```python
from build123d import *

# Parameters (mm, degrees)
SKETCH_1_W               = 135
SKETCH_1_H               = 100
EXTRUDE_1_DEPTH          = 4
SKETCH_2_W               = 135
SKETCH_2_H               = 4
EXTRUDE_2_DEPTH          = 60
CUT_EXTRUDE_1_DEPTH      = 130.12106722
CUT_EXTRUDE_1_DEPTH_BACK = 130.12106722
SKETCH_3_W               = 3
SKETCH_3_H               = 50
FILLET_1_R               = 5
FILLET_2_R               = 2
CUT_EXTRUDE_2_DEPTH      = 130.12106722
CUT_EXTRUDE_2_DEPTH_BACK = 130.12106722
SKETCH_4_R               = 1.75
CUT_EXTRUDE_3_DEPTH      = 130.12106722
CUT_EXTRUDE_3_DEPTH_BACK = 130.12106722
SKETCH_5_W               = 34
SKETCH_5_H               = 12
CUT_EXTRUDE_4_DEPTH      = 130.12106722
CUT_EXTRUDE_4_DEPTH_BACK = 130.12106722
SKETCH_6_R               = 1.75
SKETCH_7_W               = 48.5
SKETCH_7_H               = 4
CUT_EXTRUDE_5_DEPTH      = 22
CUT_EXTRUDE_6_DEPTH      = 130.12106722
CUT_EXTRUDE_6_DEPTH_BACK = 130.12106722
SKETCH_8_R               = 1.75
CUT_EXTRUDE_7_DEPTH      = 130.12106722
CUT_EXTRUDE_7_DEPTH_BACK = 130.12106722
SKETCH_9_R               = 1.75


with BuildPart() as part:
    # 草图1 → 凸台-拉伸1 (new body)
    with BuildSketch(Plane(origin=(0, 0, 0), x_dir=(1, 0, 0), z_dir=(0, 1, 0))):
        Rectangle(SKETCH_1_W, SKETCH_1_H)
    extrude(amount=EXTRUDE_1_DEPTH)

    # 草图2 → 凸台-拉伸2 (add)
    with BuildSketch(Plane.XY.offset(50)):
        with Locations((0, 2)):
            Rectangle(SKETCH_2_W, SKETCH_2_H)
    extrude(amount=EXTRUDE_2_DEPTH)

    # 草图3 → 切除-拉伸1 (cut, two sides: drawn at the far end of the back side and taken through both)
    with BuildSketch(Plane(origin=(0, 4, 0), x_dir=(1, 0, 0), z_dir=(0, 1, 0)).offset(-CUT_EXTRUDE_1_DEPTH_BACK)):
        with Locations((-66, 25)):
            Rectangle(SKETCH_3_W, SKETCH_3_H)
        with Locations((66, 25)):
            Rectangle(SKETCH_3_W, SKETCH_3_H)
        with Locations((-66, -85)):
            Rectangle(SKETCH_3_W, SKETCH_3_H)
        with Locations((66, -85)):
            Rectangle(SKETCH_3_W, SKETCH_3_H)
    extrude(amount=CUT_EXTRUDE_1_DEPTH + CUT_EXTRUDE_1_DEPTH_BACK, mode=Mode.SUBTRACT)

    # 圆角1
    fillet_1_edges = [part.edges().sort_by_distance(p)[0] for p in [
        (64.5, 2, -50),
        (-64.5, 2, 110),
        (64.5, 2, 110),
        (-64.5, 2, -50),
    ]]
    fillet(fillet_1_edges, radius=FILLET_1_R)

    # 圆角2
    fillet_2_edges = [part.edges().sort_by_distance(p)[0] for p in [
        (67.5, 2, 0),
        (-67.5, 2, 60),
        (67.5, 2, 60),
        (-67.5, 2, 0),
    ]]
    fillet(fillet_2_edges, radius=FILLET_2_R)

    # 草图4 → 切除-拉伸2 (cut, two sides: drawn at the far end of the back side and taken through both)
    with BuildSketch(Plane(origin=(0, 4, 0), x_dir=(1, 0, 0), z_dir=(0, 1, 0)).offset(-CUT_EXTRUDE_2_DEPTH_BACK)):
        with Locations(Location((-30, -102, 0), (0, 0, 270))):
            Circle(SKETCH_4_R)
        with Locations(Location((0, -102, 0), (0, 0, 270))):
            Circle(SKETCH_4_R)
        with Locations(Location((30, -102, 0), (0, 0, 270))):
            Circle(SKETCH_4_R)
        with Locations(Location((-30, 42, 0), (0, 0, 270))):
            Circle(SKETCH_4_R)
        with Locations(Location((0, 42, 0), (0, 0, 270))):
            Circle(SKETCH_4_R)
        with Locations(Location((30, 42, 0), (0, 0, 270))):
            Circle(SKETCH_4_R)
    extrude(amount=CUT_EXTRUDE_2_DEPTH + CUT_EXTRUDE_2_DEPTH_BACK, mode=Mode.SUBTRACT)

    # 草图5 → 切除-拉伸3 (cut, two sides: drawn at the far end of the back side and taken through both)
    with BuildSketch(Plane(origin=(0, 4, 0), x_dir=(1, 0, 0), z_dir=(0, 1, 0)).offset(-CUT_EXTRUDE_3_DEPTH_BACK)):
        with Locations((0, -86)):
            Rectangle(SKETCH_5_W, SKETCH_5_H)
        with Locations((0, 26)):
            Rectangle(SKETCH_5_W, SKETCH_5_H)
    extrude(amount=CUT_EXTRUDE_3_DEPTH + CUT_EXTRUDE_3_DEPTH_BACK, mode=Mode.SUBTRACT)

    # 草图6 → 切除-拉伸4 (cut, two sides: drawn at the far end of the back side and taken through both)
    with BuildSketch(Plane.XZ.offset(-CUT_EXTRUDE_4_DEPTH_BACK)):
        with Locations(Location((-16, -2, 0), (0, 0, 270))):
            Circle(SKETCH_6_R)
        with Locations(Location((16, -2, 0), (0, 0, 270))):
            Circle(SKETCH_6_R)
        with Locations(Location((16, 62, 0), (0, 0, 270))):
            Circle(SKETCH_6_R)
        with Locations(Location((-16, 62, 0), (0, 0, 270))):
            Circle(SKETCH_6_R)
    extrude(amount=CUT_EXTRUDE_4_DEPTH + CUT_EXTRUDE_4_DEPTH_BACK, mode=Mode.SUBTRACT)

    # 草图7 → 切除-拉伸5 (cut)
    with BuildSketch(Plane(origin=(0, 0, -50), x_dir=(-1, 0, 0), z_dir=(0, 0, -1))):
        with Locations((0, 2)):
            Rectangle(SKETCH_7_W, SKETCH_7_H)
    extrude(amount=-CUT_EXTRUDE_5_DEPTH, mode=Mode.SUBTRACT)

    # 草图8 → 切除-拉伸6 (cut, two sides: drawn at the far end of the back side and taken through both)
    with BuildSketch(Plane.XZ.offset(-CUT_EXTRUDE_6_DEPTH_BACK)):
        with Locations(Location((-29, -32.13, 0), (0, 0, 270))):
            Circle(SKETCH_8_R)
        with Locations(Location((29, -32.13, 0), (0, 0, 270))):
            Circle(SKETCH_8_R)
    extrude(amount=CUT_EXTRUDE_6_DEPTH + CUT_EXTRUDE_6_DEPTH_BACK, mode=Mode.SUBTRACT)

    # 草图9 → 切除-拉伸7 (cut, two sides: drawn at the far end of the back side and taken through both)
    with BuildSketch(Plane(origin=(0, 4, 0), x_dir=(1, 0, 0), z_dir=(0, 1, 0)).offset(-CUT_EXTRUDE_7_DEPTH_BACK)):
        with Locations(Location((-63, -30, 0), (0, 0, 270))):
            Circle(SKETCH_9_R)
        with Locations(Location((-63, -20, 0), (0, 0, 270))):
            Circle(SKETCH_9_R)
        with Locations(Location((-63, -10, 0), (0, 0, 270))):
            Circle(SKETCH_9_R)
        with Locations(Location((-63, -40, 0), (0, 0, 270))):
            Circle(SKETCH_9_R)
        with Locations(Location((-63, -50, 0), (0, 0, 270))):
            Circle(SKETCH_9_R)
        with Locations(Location((63, -50, 0), (0, 0, 270))):
            Circle(SKETCH_9_R)
        with Locations(Location((63, -40, 0), (0, 0, 270))):
            Circle(SKETCH_9_R)
        with Locations(Location((63, -30, 0), (0, 0, 270))):
            Circle(SKETCH_9_R)
        with Locations(Location((63, -20, 0), (0, 0, 270))):
            Circle(SKETCH_9_R)
        with Locations(Location((63, -10, 0), (0, 0, 270))):
            Circle(SKETCH_9_R)
    extrude(amount=CUT_EXTRUDE_7_DEPTH + CUT_EXTRUDE_7_DEPTH_BACK, mode=Mode.SUBTRACT)


solid = part.part
```
Could you check a few things on this model? Use its own coordinates, in mm. A direction names the side the tool comes from. Round coordinates to 2 decimals unless told otherwise and drop trailing zeros. Write each loop counter-clockwise with the first axis right and the second up, starting at its lowest first coordinate (ties: lowest second). Pieces come first, ordered by that corner, then holes. Notation, with made-up numbers: M -23.75,50.5 L -5.75,50.5 A27 ccw -5.75,76.5 Z; hole C 59,64.25 d4. An arc over 180 degrees is marked long. Answer in a Markdown table with one row per item. Add a question column.
Q1. Imagine slicing it at A-A (z = 10). Please give me the cut outline in (x, y).
Q2. Imagine slicing it at C-C (y = 3.25). Give the number of separate pieces and of enclosed holes in the cut face, then the cut area to 3 significant figures.
Q3. Will these pins go through, and if not, where does the flat tip stop? pin 1 Ø2 at (y, z) = (3.5, -11) entering from -X; pin 2 Ø2 at (x, y) = (3, 2.5) entering from -Z; pin 3 Ø10 at (x, z) = (-19, 8) entering from -Y; pin 4 Ø3 at (x, z) = (-63, 40) entering from -Y.
Q4. On a 3-axis mill with a long thin cutter (end or side, diameter ignored), from which of +Z, -Z, +X, -X, +Y, -Y can I reach the whole of each face in a straight line? I mean faces 1 (the flat face through (-17, 2, -24)), 2 (the flat face through (42, 2, -50)), 3 (the flat face through (17, 2, 86)). Say none if no direction works.
Q5. Imagine slicing it at B-B (z = 102). Please give me the cut outline in (x, y), then the cut area to 3 significant figures.
Q6. If we mould it in two halves opening along Z, with no side actions, what happens to faces 4 (the cylindrical face through (-63.07, 2.03, 108.5)), 5 (the flat face through (-67.5, 2, 30)), 6 (the flat face through (-42, 2, -50)), 7 (the cylindrical face through (-64.55, 1.97, 40.81))? For each: +Z half, -Z half, draft (parallel to the pull), parting line (faces both ways), or undercut.
Q7. If I drill on line 1 (Z direction, x = 16, y = 1.9); line 2 (X direction, y = 2, z = 10); line 3 (Z direction, x = 7, y = 1.2), over which ranges is the centre line in solid material (lowest first)? Write a range as from..to.
Q8. Imagine slicing it at D-D (z = -32.13). Please give me the cut outline in (x, y).
Values:
| question | item | result |
|---|---|---|
| 1 | outline | M -67.5,0 L -64.75,0 L -64.75,4 L -67.5,4 Z; M -61.25,0 L 61.25,0 L 61.25,4 L -61.25,4 Z; M 64.75,0 L 67.5,0 L 67.5,4 L 64.75,4 Z |
| 2 | separate pieces | 1 |
| 2 | enclosed holes | 22 |
| 2 | area | 19,000 mm^2 |
| 3 | pin 1 | x = -64.5 |
| 3 | pin 2 | z = -20 |
| 3 | pin 3 | y = 0 |
| 3 | pin 4 | through |
| 4 | face 1 | -Z, +Y, -Y |
| 4 | face 2 | -Z, +X, -X, +Y, -Y |
| 4 | face 3 | +Y, -Y |
| 5 | outline | M -64.5,0 L -31.75,0 L -31.75,4 L -64.5,4 Z; M -28.25,0 L -1.75,0 L -1.75,4 L -28.25,4 Z; M 1.75,0 L 28.25,0 L 28.25,4 L 1.75,4 Z; M 31.75,0 L 64.5,0 L 64.5,4 L 31.75,4 Z |
| 5 | area | 474 mm^2 |
| 6 | face 4 | +Z half |
| 6 | face 5 | draft |
| 6 | face 6 | -Z half |
| 6 | face 7 | undercut |
| 7 | line 1 | -20..-3.75, -0.25..60.25, 63.75..80, 92..110 |
| 7 | line 2 | -67.5..-64.75, -61.25..61.25, 64.75..67.5 |
| 7 | line 3 | -20..80, 92..110 |
| 8 | outline | M -64.5,0 L -30.75,0 L -30.75,4 L -64.5,4 Z; M -27.25,0 L -24.25,0 L -24.25,4 L -27.25,4 Z; M 24.25,0 L 27.25,0 L 27.25,4 L 24.25,4 Z; M 30.75,0 L 64.5,0 L 64.5,4 L 30.75,4 Z |
